Could you check a few things on this drawing? It's one solid part, dimensions in mm from its lowest x, y, z. Coordinates: 2 decimals unless noted, no trailing zeros. Order: outer loops, then holes, each group sorted by start corner. A loop starts at its lowest first (then second) coordinate and runs counter-clockwise, first axis right, second up.
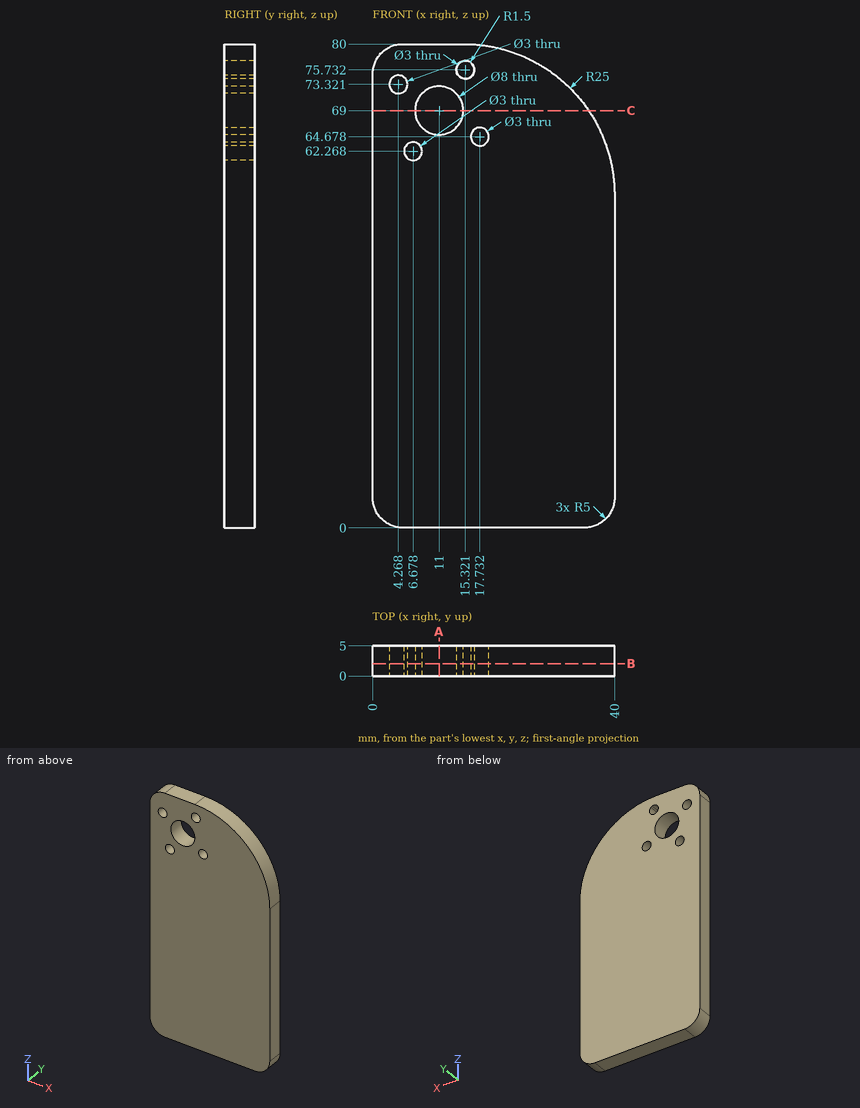
1. Please list where these lines run through material, in increasing order: probe 1 along Z at (x, y) = (11, 3.4); probe 2 along Z at (x, y) = (12.5, 3.4); probe 3 along Z at (x, y) = (33.5, 4.5) (1 decimal).
Completed:
probe 1: z = 0 to 65, 73 to 80
probe 2: z = 0 to 65.29, 72.71 to 80
probe 3: z = 0 to 71.8
2. Imagine slicing it at C-C on z = 69. Please give me the cut outline in (x, y).
Completed:
outline: (0, 0) - (7, 0) - (7, 5) - (0, 5) - close; (15, 0) - (35.71, 0) - (35.71, 5) - (15, 5) - close
3. Imagine slicing it at B-B on y = 2.05. Please give me the cut outline in (x, z).
Completed:
outline: (0, 5) arc R5 ccw to (5, 0) - (35, 0) arc R5 ccw to (40, 5) - (40, 55) arc R25 ccw to (15, 80) - (5, 80) arc R5 ccw to (0, 75) - close; hole circle Ø3 at (4.27, 73.32); hole circle Ø3 at (6.68, 62.27); hole circle Ø8 at (11, 69); hole (15.91, 77.11) arc R1.5 ccw (long way) to (16.33, 76.84) arc R1.5 ccw to start; hole circle Ø3 at (17.73, 64.68)
4. I'm going to push a flat-ended pin straight in: pin 1 (2.5 mm diameter, centred on x = 6.68, z = 62.27, fed in from -Y). Where does the tip first touch, or does it pass through?
Completed:
pin 1: passes through
5. Imagine slicing it at A-A on x = 11. Please give me the cut outline in (y, z), then the cut area to 3 significant figures.
Completed:
outline: (0, 0) - (5, 0) - (5, 65) - (0, 65) - close; (0, 73) - (5, 73) - (5, 80) - (0, 80) - close
area: 360 mm2
